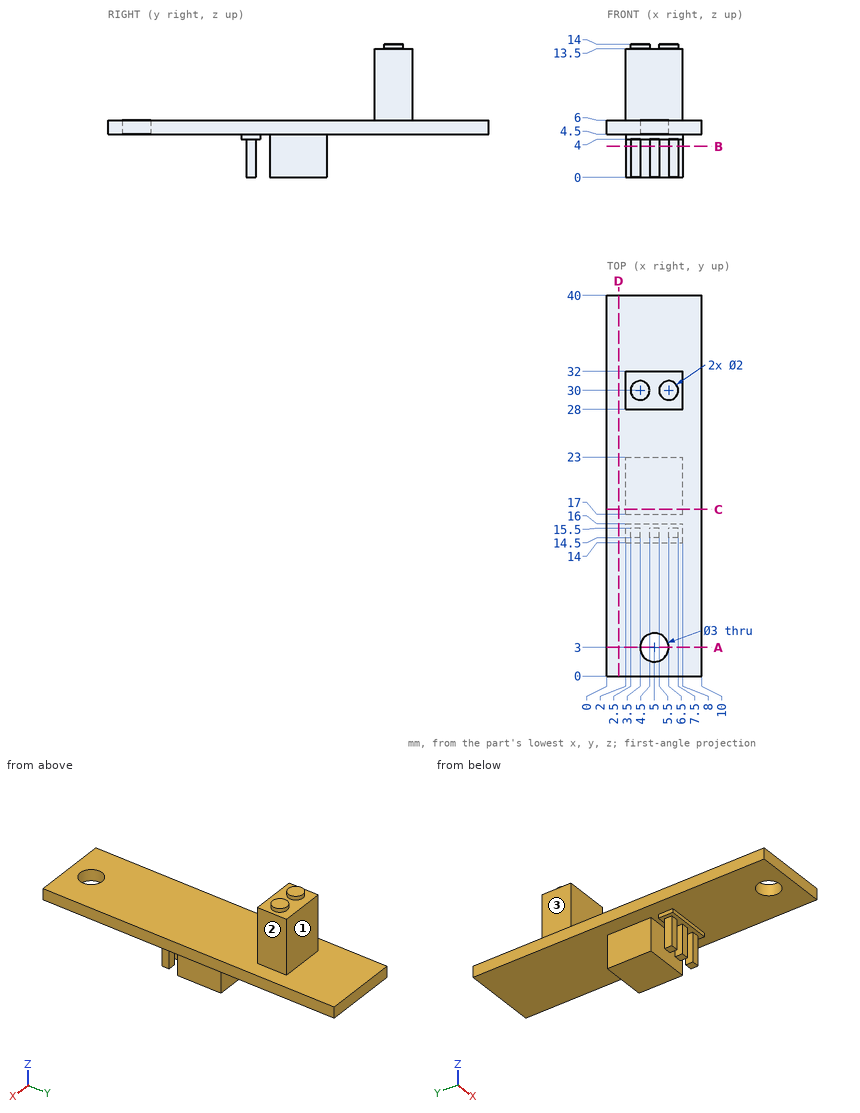
The drawing under review shows one solid part. Ordinate dimensions are in mm from its lowest x, y, z. A direction names the side the tool comes from. Coordinates: 2 decimals unless noted, no trailing zeros. Write each loop counter-clockwise with the first axis right and the second up, starting at its lowest first coordinate (ties: lowest second). Pieces come first, ordered by that corner, then holes. Notation, with made-up numbers: M -24,-19 L 35,-19 A22 ccw 35,14 Z; hole C -36,67 d3. An arc over 180 degrees is marked long. Put each result on its own line as item: value.
1) Add section C-C on y = 17.5. Give the boundary of the cut face in (x, z).
Computed:
outline: M 0,4.5 L 2,4.5 L 2,0 L 8,0 L 8,4.5 L 10,4.5 L 10,6 L 0,6 Z
2) Add section B-B on z = 3.25. Give the boundary of the cut face in (x, y).
Computed:
outline: M 2,17 L 8,17 L 8,23 L 2,23 Z; M 2.5,14.5 L 3.5,14.5 L 3.5,15.5 L 2.5,15.5 Z; M 4.5,14.5 L 5.5,14.5 L 5.5,15.5 L 4.5,15.5 Z; M 6.5,14.5 L 7.5,14.5 L 7.5,15.5 L 6.5,15.5 Z
3) Wall thickness on probe 1 along Y at (x, z) = (5, 5.2); probe 2 along Y at (x, z) = (4.75, 1); probe 3 along Z at (x, y) = (5, 34.5): over which ranges is each line inside the solid? List them lowest first. Write a range as [from, to].
Computed:
probe 1: y = [0, 1.5], [4.5, 40]
probe 2: y = [14.5, 15.5], [17, 23]
probe 3: z = [4.5, 6]
4) For the marked faces 1, 2 and 3, list the 3-axis set-ups (+Z, -Z, +X, -X, +Y, -Y) from which the entire face can be reached by the end or side of a thin tool; tool diameter is ignored.
Computed:
face 1: +Z, +X, -X, +Y
face 2: +Z, +X, +Y, -Y
face 3: +Z, -X, +Y, -Y
5) Add section D-D on x = 1.25. Give the boundary of the cut face in (y, z), then the cut area to 3 significant figures.
Computed:
outline: M 0,4.5 L 40,4.5 L 40,6 L 0,6 Z
area: 60.0 mm2
6) Clearance check with flat-ended pins moving along their axes: pin 1 Ø0.8 at (x, z) = (5, 1.5) entering from +Y; pin 2 Ø0.8 at (x, z) = (3, 1.5) entering from -Y; pin 3 Ø8 at (y, z) = (13.5, 4) entering from -X; pin 4 Ø1.5 at (x, z) = (7.5, 10) entering from -Y. State where each tip first meets the part, or that it passes through.
Computed:
pin 1: stops at y = 23
pin 2: stops at y = 14.5
pin 3: stops at x = 0
pin 4: stops at y = 28
7) Add section A-A on y = 3. Give the boundary of the cut face in (x, z), then the cut area to 3 significant figures.
Computed:
outline: M 0,4.5 L 3.5,4.5 L 3.5,6 L 0,6 Z; M 6.5,4.5 L 10,4.5 L 10,6 L 6.5,6 Z
area: 10.5 mm2
